Could you check a few things on this model? Use its own coordinates, in mm. Face numbers are marked on the shaded views. A direction names the side the tool comes from. Round coordinates to 2 decimals unless told otherwise and drop trailing zeros. Order: outer loops, then holes, each group sorted by start corner. A loop starts at its lowest first (then second) coordinate and runs counter-clockwise, first axis right, second up. Notation, with made-up numbers: (79.25, -1) - (138.25, -1) arc R26 ccw to (138.25, 26) - close; hole circle Ø2 at (6.5, -7.5). An arc over 180 degrees is marked (long way). Use one line per item in the form item = value.
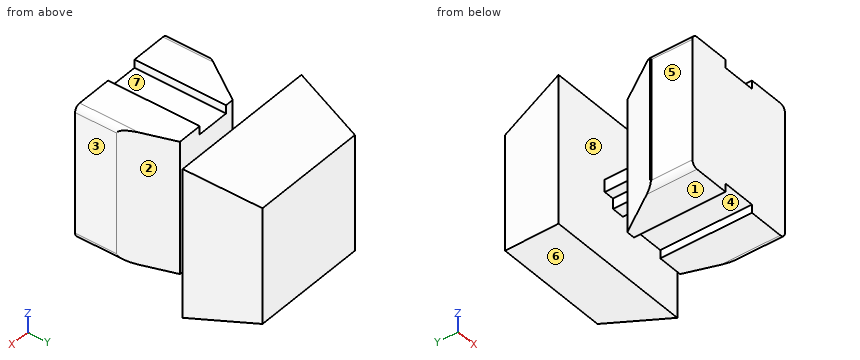
from build123d import *

# Parameters (mm, degrees)
BOSS_EXTRUDE1_DEPTH = 11
CUT_EXTRUDE1_DEPTH  = 18
CUT_EXTRUDE2_DEPTH  = 18
BOSS_EXTRUDE2_DEPTH = 3.5
BOSS_EXTRUDE3_DEPTH = 8
CUT_EXTRUDE4_DEPTH  = 27
CUT_EXTRUDE5_DEPTH  = 27
SKETCH11_W          = 14.6
SKETCH11_H          = 0.1
BOSS_EXTRUDE4_DEPTH = 0.1


with BuildPart() as part:
    # Sketch1 → Boss-Extrude1 (new body)
    with BuildSketch(Plane(origin=(0, 0, 0), x_dir=(1, 0, 0), z_dir=(0, 1, 0))):
        with BuildLine():
            Line((-6.3, -8), (-2, -8))
            Line((-2, -8), (-2, -7))
            Line((-2, -7), (2, -7))
            Line((2, -7), (2, -8))
            Line((2, -8), (6.3, -8))
            ThreePointArc((6.3, -8), (6.794974747, -7.794974747), (7, -7.3))
            Line((7, -7.3), (7, 7.3))
            ThreePointArc((7, 7.3), (6.794974747, 7.794974747), (6.3, 8))
            Line((6.3, 8), (2, 8))
            Line((2, 8), (2, 7))
            Line((2, 7), (-2, 7))
            Line((-2, 7), (-2, 8))
            Line((-2, 8), (-6.3, 8))
            ThreePointArc((-6.3, 8), (-6.794974747, 7.794974747), (-7, 7.3))
            Line((-7, 7.3), (-7, -7.3))
            ThreePointArc((-7, -7.3), (-6.794974747, -7.794974747), (-6.3, -8))
        make_face()
    extrude(amount=BOSS_EXTRUDE1_DEPTH)

    # Sketch2 → Cut-Extrude1 (cut)
    with BuildSketch(Plane.XY.offset(8)):
        Polygon((-3, 11), (-7, 5), (-7, 11), align=None)
    extrude(amount=-CUT_EXTRUDE1_DEPTH, mode=Mode.SUBTRACT)

    # Sketch3 → Cut-Extrude2 (cut)
    with BuildSketch(Plane.XY.offset(8)):
        Polygon((5, 11), (7, 5), (7, 11), align=None)
    extrude(amount=-CUT_EXTRUDE2_DEPTH, mode=Mode.SUBTRACT)

    # Sketch4 → Boss-Extrude2 (add)
    with BuildSketch(Plane(origin=(0, 11, 0), x_dir=(1, 0, 0), z_dir=(0, 1, 0))):
        Polygon((-0.75, 0.75), (-0.75, 2), (0.75, 2), (0.75, 0.75), (2, 0.75), (2, -0.75), (0.75, -0.75), (0.75, -2), (-0.75, -2), (-0.75, -0.75), (-2, -0.75), (-2, 0.75), align=None)
    extrude(amount=BOSS_EXTRUDE2_DEPTH)

    # Sketch7 → Boss-Extrude3 (add)
    with BuildSketch(Plane(origin=(0, 14.5, 0), x_dir=(1, 0, 0), z_dir=(0, 1, 0))):
        Polygon((9, -9), (-9, -9), (-9, 9), (0, 9), (9, 9), align=None)
    extrude(amount=BOSS_EXTRUDE3_DEPTH)

    # Sketch10 → Cut-Extrude4 (cut)
    with BuildSketch(Plane.ZY.offset(9)):
        Polygon((-9, 22.5), (-7, 22.5), (-9, 14.5), align=None)
        Polygon((7, 22.5), (9, 22.5), (9, 14.5), align=None)
    extrude(amount=-CUT_EXTRUDE4_DEPTH, mode=Mode.SUBTRACT)

    # Sketch8 → Cut-Extrude5 (cut)
    with BuildSketch(Plane(origin=(0, 0, -9), x_dir=(-1, 0, 0), z_dir=(0, 0, -1))):
        Polygon((9, 22.5), (7, 22.5), (9, 14.5), align=None)
        Polygon((-9, 22.5), (-7, 22.5), (-9, 14.5), align=None)
    extrude(amount=-CUT_EXTRUDE5_DEPTH, mode=Mode.SUBTRACT)

    # Sketch11 → Boss-Extrude4 (add)
    with BuildSketch(Plane.ZY.offset(7)):
        with Locations((0, 4.95)):
            Rectangle(SKETCH11_W, SKETCH11_H)
    extrude(amount=BOSS_EXTRUDE4_DEPTH)


solid = part.part
Item 1: Imagine slicing it at D-D on z = 0. Please give me the cut outline in (x, y), plus the area to 3 significant figures.
Found:
outline = (-9, 14.5) - (-2, 14.5) - (-2, 11) - (-3, 11) - (-7, 5) - (-7.1, 5) - (-7.1, 4.9) - (-7, 4.9) - (-7, 0) - (7, 0) - (7, 5) - (5, 11) - (2, 11) - (2, 14.5) - (9, 14.5) - (7, 22.5) - (-7, 22.5) - close
area = 278 mm2
Item 2: Imagine slicing it at C-C on y = 12.75. Please give me the cut outline in (x, z).
Found:
outline = (-2, -0.75) - (-0.75, -0.75) - (-0.75, -2) - (0.75, -2) - (0.75, -0.75) - (2, -0.75) - (2, 0.75) - (0.75, 0.75) - (0.75, 2) - (-0.75, 2) - (-0.75, 0.75) - (-2, 0.75) - close
Item 3: If we mould it in two halves opening along Y, with no side actions, what happens to the marked faces 6, 7 and 8? For each: released by +Y, released by -Y, zero draft, split by the parting line, or undercut.
Found:
face_6 = released by +Y
face_7 = zero draft
face_8 = undercut
Item 4: For the marked faces 1, 2, 3, 4 and 5, which set-ups out of +Z, -Z, +X, -X, +Y, -Y let a thin tool reach every point of the face, with its end or its side?
Found:
face_1 = -Z, +X, -X, -Y
face_2 = +Z, -Z, +X
face_3 = +Z, -Z, +X, -Y
face_4 = -Z, -Y
face_5 = +Z, -Z, -X, -Y
Item 5: Imagine slicing it at A-A on x = -6. Please give me the cut outline in (y, z).
Found:
outline = (0, -8) - (6.5, -8) - (6.5, 8) - (0, 8) - close; (14.5, -9) - (22.5, -7) - (22.5, 7) - (14.5, 9) - close
Item 6: I need wall thicknesses on L1, parallel to Y at x = 0.5, z = 4; L2, parallel to Z at x = -1.5, y = 8; L3, parallel to Y at x = -5, z = 3.75. Which ranges of each line are inside material? Lowest first, please.
Found:
L1 = 0 to 11, 14.5 to 22.5
L2 = -7 to 7
L3 = 0 to 8, 14.5 to 22.5
Item 7: Will these pins go through, and if not, where does the flat tip stop? P1, Ø0.8, axis at x = -0.5, y = 12.5, coming from the -Z side; P2, Ø2, axis at x = -4.5, y = 3, coming from the -Z side; P3, Ø6, axis at y = 18.5, z = 5, coming from the -X side.
Found:
P1 = -2
P2 = -8
P3 = -8.75
Item 8: Imagine slicing it at B-B on z = 5.25. Please give me the cut outline in (x, y).
Found:
outline = (-9, 14.5) - (9, 14.5) - (7, 22.5) - (-7, 22.5) - close; (-7.1, 4.9) - (-7, 4.9) - (-7, 0) - (7, 0) - (7, 5) - (5, 11) - (-3, 11) - (-7, 5) - (-7.1, 5) - close
